```python
from build123d import *

# Parameters (mm, degrees)
F2_R     = 35.907652
F2_R_2   = 18.709926
F3_DEPTH = 3.95508
F4_R     = 2.749
F5_DEPTH = 47


with BuildPart() as f1:
    # F0 (on Front) → F1 (revolve)
    with BuildSketch(Plane.XZ):
        Polygon((-56.319889, 0), (-51.850058, 0), (-51.850058, 10.876591), (0, 10.876591), (0, 48.423186), (-15.793407, 48.423186), (-12.515531, 44.251341), (-19.667262, 34.119722), (-46.486259, 34.119722), (-46.486259, 16.53838), (-56.319889, 16.53838), align=None)
    revolve(axis=Axis((-0.162292, 0, 0), (1, 0, 0)))

    # F2 (on face) → F3 (cut)
    with BuildSketch(Plane.YZ):
        Circle(F2_R)
        Circle(F2_R_2, mode=Mode.SUBTRACT)
    extrude(amount=-F3_DEPTH, mode=Mode.SUBTRACT)

    # F4 (on face) → F5 (cut)
    with BuildSketch(Plane.YZ.offset(-3.95508)):
        with Locations((0, 25.776034)):
            Circle(F4_R)
        with Locations((-9.864061, 23.81395)):
            Circle(F4_R)
        with Locations((-18.226409, 18.226409)):
            Circle(F4_R)
        with Locations((-23.81395, 9.864061)):
            Circle(F4_R)
        with Locations((-25.776034, 0)):
            Circle(F4_R)
        with Locations((-23.81395, -9.864061)):
            Circle(F4_R)
        with Locations((-18.226409, -18.226409)):
            Circle(F4_R)
        with Locations((-9.864061, -23.81395)):
            Circle(F4_R)
        with Locations((0, -25.776034)):
            Circle(F4_R)
        with Locations((9.864061, -23.81395)):
            Circle(F4_R)
        with Locations((18.226409, -18.226409)):
            Circle(F4_R)
        with Locations((23.81395, -9.864061)):
            Circle(F4_R)
        with Locations((25.776034, 0)):
            Circle(F4_R)
        with Locations((23.81395, 9.864061)):
            Circle(F4_R)
        with Locations((18.226409, 18.226409)):
            Circle(F4_R)
        with Locations((9.864061, 23.81395)):
            Circle(F4_R)
    extrude(amount=-F5_DEPTH, mode=Mode.SUBTRACT)


solid = f1.part
```
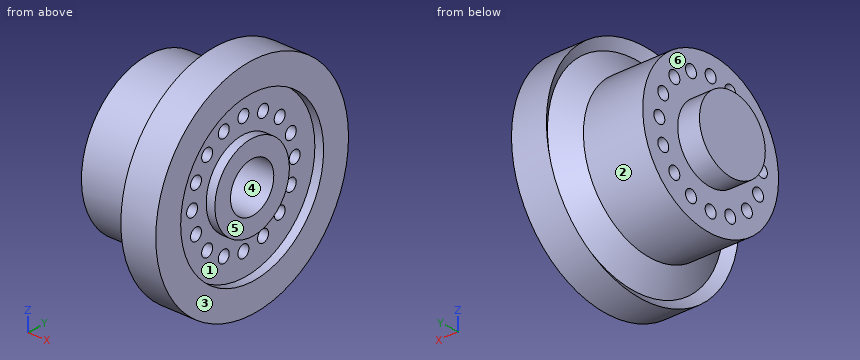
The model under review builds one solid part; all positions refer to its coordinate system, in mm. Face numbers are marked on the shaded views. A direction names the side the tool comes from. Give positions to 0.01 mm unless a question says otherwise; leave off trailing zeros.
(1) For P1, Ø6.5, axis at y = 18.23, z = -18.23, coming from the -X side; P2, Ø3.5, axis at y = 9.86, z = 23.81, coming from the +X side; P3, Ø2, axis at x = -28, y = 12.5, coming from the -Z side; P4, Ø7, axis at y = 23.81, z = 9.86, coming from the +X side, all flat-tipped, find the tip position at first contact; note any pin that passes through.
(2) Consider section A-A, the plane y = 0. Give the number of separate pieces and of enclosed holes in the cut face, and give its area (3 significant figures).
(3) The part is to be moulded in two halves that separate along Z. For the marked faces 1, 2 and 3, say which applies: released by +Z, released by -Z, zero draft, split by the parting line, or undercut.
(4) Tool access review of the marked faces 4, 5 and 6: name each direction out of +Z, -Z, +X, -X, +Y, -Y from which nothing blocks a thin tool from reaching the whole face with its end or side.
(5) To check wall thickness, follow L1, parallel to Z at x = -27.5, y = 0; L2, parallel to Y at x = -8, z = 1.5; L3, parallel to Y at x = -28.5, z = -24. State the ranges of each line that lie inside material, in increasing order.
Returned:
1. P1: stops at x = -46.49
1. P2: passes through
1. P3: stops at z = -32.12
1. P4: stops at x = -3.96
2. separate pieces: 3
2. enclosed holes: 0
2. area: 2,210 mm2
3. face 1: undercut
3. face 2: split by the parting line
3. face 3: zero draft
4. face 4: +X
4. face 5: +Z, -Z, +X, +Y, -Y
4. face 6: -X
5. L1: z = -34.12 to -28.53, -23.03 to -10.88, 10.88 to 23.03, 28.53 to 34.12
5. L2: y = -48.4 to -28.08, -23.47 to -10.77, 10.77 to 23.47, 28.08 to 48.4
5. L3: y = -24.25 to -12.61, -7.12 to -2.1, 2.1 to 7.12, 12.61 to 24.25
